from build123d import *

# Parameters (mm, degrees)
SKETCH1_W           = 25.4
SKETCH1_H           = 25.4
BOSS_EXTRUDE1_DEPTH = 25.4
SKETCH2_W           = 3.175
SKETCH2_H           = 15.875
BOSS_EXTRUDE2_DEPTH = 15.875
BOSS_EXTRUDE3_DEPTH = 2.54
SKETCH8_R           = 3.175
CUT_EXTRUDE1_DEPTH  = 54.317316605
FILLET1_R           = 0.6
SKETCH9_W           = 24.2
SKETCH9_H           = 24.2
BOSS_EXTRUDE4_DEPTH = 12.7


with BuildPart() as part:
    # Sketch1 → Boss-Extrude1 (new body)
    with BuildSketch(Plane.XY):
        with Locations((-12.7, 12.7)):
            Rectangle(SKETCH1_W, SKETCH1_H)
    extrude(amount=BOSS_EXTRUDE1_DEPTH)

    # Sketch2 → Boss-Extrude2 (add)
    with BuildSketch(Plane(origin=(0, 25.4, 0), x_dir=(1, 0, 0), z_dir=(0, 1, 0))):
        with Locations((-1.5875, -12.7)):
            Rectangle(SKETCH2_W, SKETCH2_H)
    extrude(amount=BOSS_EXTRUDE2_DEPTH)

    # Sketch6 → Boss-Extrude3 (add)
    with BuildSketch(Plane.XY.offset(20.6375)):
        Polygon((-3.175, 25.4), (-6.35, 25.4), (-3.175, 31.75), align=None)
    boss_extrude3 = extrude(amount=-BOSS_EXTRUDE3_DEPTH)

    # Mirror1: Boss-Extrude3 across plane
    add(boss_extrude3.mirror(Plane.XY.offset(12.7)))

    # Sketch8 → Cut-Extrude1 (cut, through all)
    with BuildSketch(Plane.ZY.offset(3.175)):
        with Locations(Location((12.7, 34.925, 0), (0, 0, 270))):
            Circle(SKETCH8_R)
    extrude(amount=-CUT_EXTRUDE1_DEPTH, mode=Mode.SUBTRACT)

    # Fillet1
    fillet1_edges = [part.edges().sort_by_distance(p)[0] for p in [
        (-12.7, 25.4, 25.4),
        (0, 12.7, 25.4),
        (-25.4, 25.4, 12.7),
        (-25.4, 12.7, 25.4),
        (-12.7, 25.4, 0),
        (-25.4, 12.7, 0),
        (0, 12.7, 0),
        (-25.4, 0, 12.7),
        (-12.7, 0, 25.4),
        (0, 0, 12.7),
        (-12.7, 0, 0),
        (0, 25.4, 23.01875),
        (0, 25.4, 2.38125),
    ]]
    fillet(fillet1_edges, radius=FILLET1_R)

    # Sketch9 → Boss-Extrude4 (add)
    with BuildSketch(Plane(origin=(0, 0, 0), x_dir=(-1, 0, 0), z_dir=(0, -1, 0))):
        with Locations((12.7, -12.7)):
            Rectangle(SKETCH9_W, SKETCH9_H)
    extrude(amount=BOSS_EXTRUDE4_DEPTH)


solid = part.part
The listing builds one solid part. Answer for the finished solid, in the listing's coordinates (mm). A direction names the side the tool comes from. Give positions to 0.01 mm unless a question says otherwise; leave off trailing zeros. Write each loop counter-clockwise with the first axis right and the second up, starting at its lowest first coordinate (ties: lowest second). Pieces come first, ordered by that corner, then holes. Notation, with made-up numbers: (55, 57) -> (60, 57) arc R15 ccw to (60, 64) -> close; hole circle Ø3 at (-7.75, -30). An arc over 180 degrees is marked (long way). One line per question, with ' | ' between items. Start each with the question number.
1. For a pull along Z with two mould halves and no side action, classify faces 1 (the flat face through (-3.175, 31, 13)), 2 (the flat face through (-2, 33, 20.638)), 3 (the flat face through (-2, 41.275, 13)) as pulls with the +Z half, pulls with the -Z half, needs draft (parallel to the pull), parting line crosses it, or undercut.
2. For faces 4 (the flat face through (-24.8, -6, 13)), 5 (the flat face through (-4, 27, 18.098)), 6 (the flat face through (-0.6, -6, 13)), 7 (the flat face through (-13, -6, 24.8)), determine the directions among +Z, -Z, +X, -X, +Y, -Y from which every point of the face is accessible in a straight line to the end or side of a thin tool.
3. Section D-D (x = -20) is taken. Determine the outline of the cut face in (y, z).
4. Section A-A (z = 12.7) is taken. Determine the outline of the cut face in (x, y) (3 decimals).
5. Given pin 1 Ø5 at (x, z) = (-17.5, 16.5) entering from +Y; pin 2 Ø3 at (x, y) = (-5, 31) entering from -Z; pin 3 Ø10 at (y, z) = (-9, 18.5) entering from -X; pin 4 Ø5.5 at (y, z) = (34.925, 12.7) entering from +X, each flat-ended and moving along its own axis, determine where each tip first touches the part or whether it passes through.
6. Section C-C (y = 33) is taken. Determine the outline of the cut face in (x, z) (1 decimal), plus the area to 3 significant figures.
7. Find the intervals of material crossed by probe 1 along X at (y, z) = (-10, 21); probe 2 along Y at (x, z) = (-18.5, 1.25); probe 3 along X at (y, z) = (35.5, 16) (3 decimals), in increasing order.
Response values:
1) face 1: undercut | face 2: pulls with the +Z half | face 3: needs draft
2) face 4: +Z, -Z, -X, -Y | face 5: -X, +Y | face 6: +Z, -Z, +X, -Y | face 7: +Z, +X, -X, -Y
3) outline: (-12.7, 0.6) -> (0, 0.6) arc R0.6 ccw to (0.6, 0) -> (24.8, 0) arc R0.6 ccw to (25.4, 0.6) -> (25.4, 24.8) arc R0.6 ccw to (24.8, 25.4) -> (0.6, 25.4) arc R0.6 ccw to (0, 24.8) -> (-12.7, 24.8) -> close
4) outline: (-25.4, 0.6) arc R0.6 ccw to (-24.8, 0) -> (-24.8, -12.7) -> (-0.6, -12.7) -> (-0.6, 0) arc R0.6 ccw to (0, 0.6) -> (0, 31.75) -> (-3.175, 31.75) -> (-3.175, 25.4) -> (-24.8, 25.4) arc R0.6 ccw to (-25.4, 24.8) -> close; (-3.175, 38.1) -> (0, 38.1) -> (0, 41.275) -> (-3.175, 41.275) -> close
5) pin 1: y = 25.4 | pin 2: z = 4.76 | pin 3: x = -24.8 | pin 4: through
6) outline: (-3.2, 4.8) -> (0, 4.8) -> (0, 10.2) -> (-3.2, 10.2) -> close; (-3.2, 15.2) -> (0, 15.2) -> (0, 20.6) -> (-3.2, 20.6) -> close | area: 34.4 mm2
7) probe 1: -24.8 to -0.6 | probe 2: -12.7 to 25.4 | probe 3: -3.175 to 0
